```python
from build123d import *

# Parameters (mm, degrees)
SKETCH1_W           = 15.24
SKETCH1_H           = 10.16
BOSS_EXTRUDE1_DEPTH = 4
SKETCH2_R           = 3.81
CUT_EXTRUDE1_DEPTH  = 3
BOSS_EXTRUDE2_DEPTH = 10.16


with BuildPart() as part:
    # Sketch1 → Boss-Extrude1 (new body)
    with BuildSketch(Plane(origin=(0, 0, 0), x_dir=(1, 0, 0), z_dir=(0, 1, 0))):
        Rectangle(SKETCH1_W, SKETCH1_H)
    extrude(amount=BOSS_EXTRUDE1_DEPTH)

    # Sketch2 → Cut-Extrude1 (cut)
    with BuildSketch(Plane(origin=(0, 4, 0), x_dir=(1, 0, 0), z_dir=(0, 1, 0))):
        Circle(SKETCH2_R)
    extrude(amount=-CUT_EXTRUDE1_DEPTH, mode=Mode.SUBTRACT)

    # Sketch3 → Boss-Extrude2 (add)
    with BuildSketch(Plane.XY.offset(5.08)):
        with BuildLine():
            Line((13.62, 4), (7.62, 4))
            Line((7.62, 4), (7.62, 0))
            Line((7.62, 0), (13.62, 0))
            ThreePointArc((13.62, 0), (28.319939798, -4.147298344), (41.51503945, -11.84))
            Line((41.51503945, -11.84), (46.73503945, -11.84))
            ThreePointArc((46.73503945, -11.84), (31.406388408, -1.350932139), (13.62, 4))
        make_face()
        with BuildLine():
            ThreePointArc((-13.62, 4), (-31.406388408, -1.350932139), (-46.73503945, -11.84))
            Line((-46.73503945, -11.84), (-41.51503945, -11.84))
            ThreePointArc((-41.51503945, -11.84), (-28.319939798, -4.147298344), (-13.62, 0))
            Line((-13.62, 0), (-7.62, 0))
            Line((-7.62, 0), (-7.62, 4))
            Line((-7.62, 4), (-13.62, 4))
        make_face()
    extrude(amount=-BOSS_EXTRUDE2_DEPTH)


solid = part.part
```
Work out the finished part from the listing and answer in its coordinate system (mm). A direction names the side the tool comes from. Coordinates: 2 decimals unless noted, no trailing zeros. Loops run counter-clockwise (first coordinate to the right, second up) from the corner with the lowest first, then second, coordinate; pieces in that order, holes last.
1) Consider probe 1 along Z at (x, y) = (0, 2.85); probe 2 along Y at (x, z) = (3, -2.5); probe 3 along X at (y, z) = (-7, -3.5). Determine where each line is inside the solid, lowest interval first.
Results:
probe 1: z = -5.08 to -3.81, 3.81 to 5.08
probe 2: y = 0 to 4
probe 3: x = -40.89 to -34.15, 34.15 to 40.89
2) Section C-C (y = -10.25) is taken. Give the vertices of the cut face in (x, z).
Results:
outline: (-44.97, -5.08) - (-39.34, -5.08) - (-39.34, 5.08) - (-44.97, 5.08) - close; (39.34, -5.08) - (44.97, -5.08) - (44.97, 5.08) - (39.34, 5.08) - close
3) Section A-A (x = 0) is taken. Give the vertices of the cut face in (y, z).
Results:
outline: (0, -5.08) - (4, -5.08) - (4, -3.81) - (1, -3.81) - (1, 3.81) - (4, 3.81) - (4, 5.08) - (0, 5.08) - close
4) Section D-D (y = 2) is taken. Give the vertices of the cut face in (x, z), plus the area to 3 significant figures.
Results:
outline: (-22.75, -5.08) - (22.75, -5.08) - (22.75, 5.08) - (-22.75, 5.08) - close; hole circle Ø7.62 at (0, 0)
area: 417 mm2
5) Flat-ended cylindrical pins translate along their axes: pin 1 (6 mm diameter, centred on x = 1.5, z = 0.5, fed in from +Y); pin 2 (3 mm diameter, centred on x = -32, z = -4, fed in from +Y); pin 3 (1 mm diameter, centred on x = -29.5, z = 0.5, fed in from +Y); pin 4 (1.5 mm diameter, centred on y = -3.5, z = 1.5, fed in from -X). Find the tip coordinate at first contact, or state that the pin passes through.
Results:
pin 1: stops at y = 4
pin 2: stops at y = -0.93
pin 3: stops at y = -0.26
pin 4: stops at x = -36.76
6) For a pull along Z with two mould halves and no side action, classify faces 4 (the flat face through (0, 1, 5.08)), 5 (the flat face through (0, 1, 0)), 6 (the cylindrical face through (28.122, -4.064, 0.071)), 7 (the flat face through (0, 1, -5.08)) as +Z half, -Z half, draft (parallel to the pull), parting line (faces both ways), or undercut.
Results:
face 4: +Z half
face 5: undercut
face 6: draft
face 7: -Z half
7) Section B-B (z = 0) is taken. Give the vertices of the cut face in (x, y).
Results:
outline: (-46.74, -11.84) - (-41.52, -11.84) arc R60.57 cw to (-13.62, 0) - (13.62, 0) arc R60.57 cw to (41.52, -11.84) - (46.74, -11.84) arc R60.57 ccw to (13.62, 4) - (3.81, 4) - (3.81, 1) - (-3.81, 1) - (-3.81, 4) - (-13.62, 4) arc R60.57 ccw to start
8) For faces 1 (the cylindrical face through (-31.17, -1.24, 0.07)), 2 (the flat face through (0, 0, 0)), 3 (the cylindrical face through (-0.83, 2.52, 3.72)), determine the directions among +Z, -Z, +X, -X, +Y, -Y from which every point of the face is accessible in a straight line to the end or side of a thin tool.
Results:
face 1: +Z, -Z, -X, +Y
face 2: +Z, -Z, -Y
face 3: +Y
